CAD build for the part. Positions are in the model's coordinates, mm. Face numbers are marked on the shaded views. A direction names the side the tool comes from. Round coordinates to 2 decimals unless told otherwise and drop trailing zeros. Loops run counter-clockwise (first coordinate to the right, second up) from the corner with the lowest first, then second, coordinate; pieces in that order, holes last. Notation, with made-up numbers: M -1,75 L 41,75 A14 ccw 41,92 Z; hole C -14,-34.5 d1. An arc over 180 degrees is marked long. Put each result on its own line as item: value. Start each with the question number.
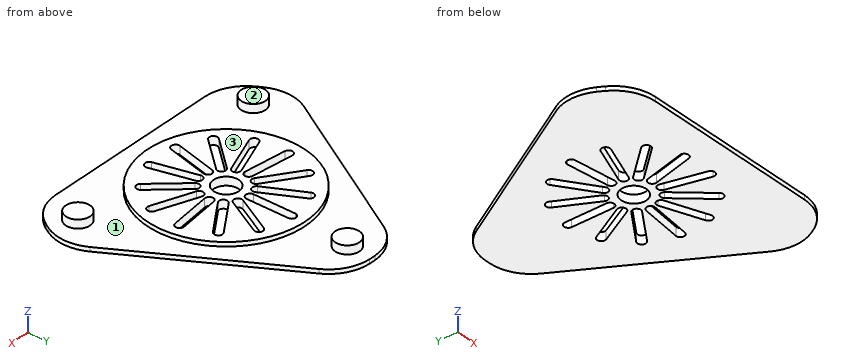
from build123d import *

# Parameters (mm, degrees)
SKETCH2_R           = 18.85
SKETCH2_R_2         = 3
BOSS_EXTRUDE1_DEPTH = 2
BOSS_EXTRUDE2_START = -1
SKETCH3_R           = 35
SKETCH3_R_2         = 18.85
BOSS_EXTRUDE2_DEPTH = 1
SKETCH4_R           = 2.9
BOSS_EXTRUDE3_DEPTH = 3
SKETCH6_R           = 5
BOSS_EXTRUDE4_DEPTH = 1
SKETCH7_R           = 59.131365533
CUT_EXTRUDE1_DEPTH  = 10
FILLET1_R           = 10


with BuildPart() as part:
    # Sketch2 → Boss-Extrude1 (new body)
    with BuildSketch(Plane.XY.offset(10)):
        Circle(SKETCH2_R)
        Circle(SKETCH2_R_2, mode=Mode.SUBTRACT)
        with BuildLine():
            Line((1, 15.711728477), (1, 5.711728477))
            ThreePointArc((1, 5.711728477), (0, 4.711728477), (-1, 5.711728477))
            Line((-1, 5.711728477), (-1, 15.711728477))
            ThreePointArc((-1, 15.711728477), (0, 16.711728477), (1, 15.711728477))
        make_face(mode=Mode.SUBTRACT)
        with BuildLine():
            Line((6.416148271, 14.376767826), (1.76891655, 5.522207569))
            ThreePointArc((1.76891655, 5.522207569), (2.189649404, 4.172028372), (3.539828602, 4.592761225))
            Line((3.539828602, 4.592761225), (8.187060322, 13.447321482))
            ThreePointArc((8.187060322, 13.447321482), (7.766327468, 14.797500679), (6.416148271, 14.376767826))
        make_face(mode=Mode.SUBTRACT)
        with BuildLine():
            Line((12.362434295, 9.748262924), (4.132595637, 4.067615457))
            ThreePointArc((4.132595637, 4.067615457), (3.877676517, 2.676566844), (5.26872513, 2.421647725))
            Line((5.26872513, 2.421647725), (13.498563789, 8.102295192))
            ThreePointArc((13.498563789, 8.102295192), (13.753482908, 9.493343805), (12.362434295, 9.748262924))
        make_face(mode=Mode.SUBTRACT)
        with BuildLine():
            Line((15.476635607, 2.886548466), (5.549546866, 1.681181663))
            ThreePointArc((5.549546866, 1.681181663), (4.677374672, 0.567936109), (5.790620226, -0.304236085))
            Line((5.790620226, -0.304236085), (15.717708967, 0.901130718))
            ThreePointArc((15.717708967, 0.901130718), (16.589881161, 2.014376272), (15.476635607, 2.886548466))
        make_face(mode=Mode.SUBTRACT)
        with BuildLine():
            Line((15.045326214, -4.636439459), (5.695163787, -1.090390589))
            ThreePointArc((5.695163787, -1.090390589), (4.405542658, -1.670801945), (4.985954013, -2.960423074))
            Line((4.985954013, -2.960423074), (14.33611644, -6.506471945))
            ThreePointArc((14.33611644, -6.506471945), (15.62573757, -5.926060589), (15.045326214, -4.636439459))
        make_face(mode=Mode.SUBTRACT)
        with BuildLine():
            Line((11.167313902, -11.097274979), (4.536087319, -3.612167498))
            ThreePointArc((4.536087319, -3.612167498), (3.124453913, -3.526779408), (3.039065823, -4.938412814))
            Line((3.039065823, -4.938412814), (9.670292405, -12.423520296))
            ThreePointArc((9.670292405, -12.423520296), (11.081925812, -12.508908386), (11.167313902, -11.097274979))
        make_face(mode=Mode.SUBTRACT)
        with BuildLine():
            Line((4.731004555, -15.015858538), (2.337847912, -5.306440364))
            ThreePointArc((2.337847912, -5.306440364), (1.127590431, -4.574814211), (0.395964277, -5.785071693))
            Line((0.395964277, -5.785071693), (2.78912092, -15.494489867))
            ThreePointArc((2.78912092, -15.494489867), (3.999378402, -16.22611602), (4.731004555, -15.015858538))
        make_face(mode=Mode.SUBTRACT)
        with BuildLine():
            Line((-2.78912092, -15.494489867), (-0.395964277, -5.785071693))
            ThreePointArc((-0.395964277, -5.785071693), (-1.127590431, -4.574814211), (-2.337847912, -5.306440364))
            Line((-2.337847912, -5.306440364), (-4.731004555, -15.015858538))
            ThreePointArc((-4.731004555, -15.015858538), (-3.999378402, -16.22611602), (-2.78912092, -15.494489867))
        make_face(mode=Mode.SUBTRACT)
        with BuildLine():
            Line((-9.670292405, -12.423520296), (-3.039065823, -4.938412814))
            ThreePointArc((-3.039065823, -4.938412814), (-3.124453913, -3.526779408), (-4.536087319, -3.612167498))
            Line((-4.536087319, -3.612167498), (-11.167313902, -11.097274979))
            ThreePointArc((-11.167313902, -11.097274979), (-11.081925812, -12.508908386), (-9.670292405, -12.423520296))
        make_face(mode=Mode.SUBTRACT)
        with BuildLine():
            Line((-14.33611644, -6.506471945), (-4.985954013, -2.960423074))
            ThreePointArc((-4.985954013, -2.960423074), (-4.405542658, -1.670801945), (-5.695163787, -1.090390589))
            Line((-5.695163787, -1.090390589), (-15.045326214, -4.636439459))
            ThreePointArc((-15.045326214, -4.636439459), (-15.62573757, -5.926060589), (-14.33611644, -6.506471945))
        make_face(mode=Mode.SUBTRACT)
        with BuildLine():
            Line((-15.717708967, 0.901130718), (-5.790620226, -0.304236085))
            ThreePointArc((-5.790620226, -0.304236085), (-4.677374672, 0.567936109), (-5.549546866, 1.681181663))
            Line((-5.549546866, 1.681181663), (-15.476635607, 2.886548466))
            ThreePointArc((-15.476635607, 2.886548466), (-16.589881161, 2.014376272), (-15.717708967, 0.901130718))
        make_face(mode=Mode.SUBTRACT)
        with BuildLine():
            Line((-13.498563789, 8.102295192), (-5.26872513, 2.421647725))
            ThreePointArc((-5.26872513, 2.421647725), (-3.877676517, 2.676566844), (-4.132595637, 4.067615457))
            Line((-4.132595637, 4.067615457), (-12.362434295, 9.748262924))
            ThreePointArc((-12.362434295, 9.748262924), (-13.753482908, 9.493343805), (-13.498563789, 8.102295192))
        make_face(mode=Mode.SUBTRACT)
        with BuildLine():
            Line((-8.187060322, 13.447321482), (-3.539828602, 4.592761225))
            ThreePointArc((-3.539828602, 4.592761225), (-2.189649404, 4.172028372), (-1.76891655, 5.522207569))
            Line((-1.76891655, 5.522207569), (-6.416148271, 14.376767826))
            ThreePointArc((-6.416148271, 14.376767826), (-7.766327468, 14.797500679), (-8.187060322, 13.447321482))
        make_face(mode=Mode.SUBTRACT)
    extrude(amount=-BOSS_EXTRUDE1_DEPTH)

    # Sketch3 → Boss-Extrude2 (add)
    with BuildSketch(Plane(origin=(0, 0, 8), x_dir=(-1, 0, 0), z_dir=(0, 0, -1)).offset(BOSS_EXTRUDE2_START)):
        Circle(SKETCH3_R)
        with Locations(Location((0, 0, 0), (0, 0, 180))):
            Circle(SKETCH3_R_2, mode=Mode.SUBTRACT)
    extrude(amount=BOSS_EXTRUDE2_DEPTH)

    # Sketch4 → Boss-Extrude3 (add)
    with BuildSketch(Plane(origin=(0, 0, 8), x_dir=(-1, 0, 0), z_dir=(0, 0, -1))):
        with Locations((0, 29)):
            Circle(SKETCH4_R)
        with Locations((25.11473671, -14.5)):
            Circle(SKETCH4_R)
        with Locations((-25.11473671, -14.5)):
            Circle(SKETCH4_R)
    extrude(amount=-BOSS_EXTRUDE3_DEPTH)

    # Sketch6 → Boss-Extrude4 (add)
    with BuildSketch(Plane(origin=(0, 0, 9), x_dir=(-1, 0, 0), z_dir=(0, 0, -1))):
        with Locations((0, 30)):
            Circle(SKETCH6_R)
        with Locations((25.980762114, -15)):
            Circle(SKETCH6_R)
        with Locations((-25.980762114, -15)):
            Circle(SKETCH6_R)
    extrude(amount=BOSS_EXTRUDE4_DEPTH)

    # Sketch7 → Cut-Extrude1 (cut)
    with BuildSketch(Plane(origin=(0, 0, 8), x_dir=(-1, 0, 0), z_dir=(0, 0, -1))):
        Circle(SKETCH7_R)
        Polygon((0, 46), (-39.837168574, -23), (39.837168574, -23), align=None, mode=Mode.SUBTRACT)
    extrude(amount=-CUT_EXTRUDE1_DEPTH, mode=Mode.SUBTRACT)

    # Fillet1
    fillet1_edges = [part.edges().sort_by_distance(p)[0] for p in [
        (-6.727678329, 34.347319318, 8.5),
        (-33.109490245, -11.347319318, 8.5),
        (-26.381811917, -23, 8.5),
        (26.381811917, -23, 8.5),
        (33.109490245, -11.347319318, 8.5),
        (6.727678329, 34.347319318, 8.5),
    ]]
    fillet(fillet1_edges, radius=FILLET1_R)


solid = part.part
(1) Drill centre lines: line 1 along Y through (x, z) = (0, 8.5); line 2 along Y through (x, z) = (0, 9.05); line 3 along Y through (x, z) = (13, 8.55). Where is each one in solid material? Low to high.
(2) Cut at A-A on z = 9.5. Count the separate pieces of the cut face and the enclosed holes in it, and give its area (3 significant figures).
(3) Cut at C-C on y = 29. List the corners of the cut face in (x, z).
(4) Tool access for the marked faces 1, 2 and 3: list every direction of +Z, -Z, +X, -X, +Y, -Y with a clear straight run to the whole face (end or side of a thin tool).
(5) Flat gauge pins, fed straight in: pin 1 Ø3.5 at (x, y) = (0, 0) entering from -Z; pin 2 Ø1.5 at (x, y) = (-15.5, -13) entering from +Z; pin 3 Ø17.5 at (x, y) = (-4.5, 2.5) entering from +Z. Where does each tip first touch, or does it go through?
(6) Cut at B-B on x = 24. List the corners of the cut face in (y, z), and give its area (3 significant figures).
Taken from the geometry:
1. line 1: -23 to -3, 3 to 4.71, 16.71 to 35
1. line 2: -18.85 to -3, 3 to 4.71, 16.71 to 18.85, 26.1 to 31.9
1. line 3: -23 to -6, -3.86 to 0.57, 2.59 to 7.76, 9.92 to 23.48
2. separate pieces: 4
2. enclosed holes: 14
2. area: 866 mm2
3. outline: M -9.81,8 L 9.81,8 L 9.81,9 L 2.9,9 L 2.9,11 L -2.9,11 L -2.9,9 L -9.81,9 Z
4. face 1: +Z
4. face 2: +Z, +X, -X, +Y, -Y
4. face 3: +Z, -Y
5. pin 1: through
5. pin 2: z = 9
5. pin 3: z = 10
6. outline: M -22.64,8 L 4.43,8 L 4.43,9 L -11.82,9 L -11.82,11 L -17.18,11 L -17.18,9 L -22.64,9 Z
6. area: 37.8 mm2
